Source: CAD feature listing. Evaluate the final solid. Frame: model axes, mm. A direction names the side the tool comes from. Give positions to 0.01 mm unless a question says otherwise; leave off trailing zeros. Loops run counter-clockwise (first coordinate to the right, second up) from the corner with the lowest first, then second, coordinate; pieces in that order, holes last. Notation, with made-up numbers: (-9, 50.25) - (3, 50.25) arc R21 ccw to (3, 85.25) - close; hole circle Ø11 at (87, -5.75). An arc over 180 degrees is marked (long way). Write each question's results on one line, items separated by ' | '. Start each with the question number.
(1) Contact query for flat-ended pins moving along their axis: pin 1 (5 mm diameter, centred on x = 3, z = -28, fed in from +Y); pin 2 (3 mm diameter, centred on y = -3, z = -29.5, fed in from +X); pin 3 (4 mm diameter, centred on y = -2, z = 7.5, fed in from +X); pin 4 (2 mm diameter, centred on x = -26.5, z = -17.5, fed in from +Y). Output: stop coordinate, or through.
(2) Pull-direction query (X, two-part tool) for faces 1 (the flat face through (11, -11, -29)), 2 (the cylindrical face through (-5.08, -7.6, -3.89)), 3 (the flat face through (-8.534, -17.535, 5.019)), 4 (the cylindrical face through (-8.67, -6.9, -39.05)); classes: pulls with the +X half, pulls with the -X half, needs draft (parallel to the pull), parting line crosses it, or undercut.
(3) Material intervals for line 1 along Z through (x, y) = (0, -5.25); line 2 along Z through (x, y) = (-1.5, -3.25); line 3 along X through (y, z) = (-9.5, -32), sorted ascending. Write a range as [from, to].
(4) Cut plane B-B on y = -10. Return the cut outline in (x, z), then the cut area to 3 significant figures.
(5) Reachability of faces 5 (the flat face through (-1, 0, -8)), 6 (the flat face through (11, -6, 24)), 7 (the flat face through (0, -18, -9.9)) from +Z, -Z, +X, -X, +Y, -Y: full face, straight path, thin tool, end or side. Return the list, or none.
(6) Cut plane A-A on x = 0. Return the cut outline in (y, z), then the cut area to 3 significant figures.
from build123d import *

# Parameters (mm, degrees)
F0_R          = 40
F1_DEPTH      = 20
F2_W          = 11
F2_H          = 10
F3_DEPTH      = 50
F3_DEPTH_BACK = 10
F4_R          = 6
F6_DEPTH      = 5
F7_R          = 6.4
F8_DEPTH      = 25


# Not quite as in the source:
# - a pattern or mirror of a feature is missing from the dataset's text; its kind, count and spacing are read off the source's solid


with BuildPart() as f1:
    # F0 (on Front) → F1 (new body)
    with BuildSketch(Plane.XZ):
        Circle(F0_R)
    extrude(amount=F1_DEPTH)

    # F2 (on Right) → F3 (cut, two sides)
    with BuildSketch(Plane.YZ) as f3_sk:
        with Locations((-5.5, 29)):
            Rectangle(F2_W, F2_H)
    f3 = extrude(amount=F3_DEPTH, mode=Mode.SUBTRACT) + extrude(f3_sk.sketch, amount=-F3_DEPTH_BACK, mode=Mode.SUBTRACT)

    # F3_copies: F3 across plane
    add(f3.mirror(Plane(origin=(0, 0, 0), x_dir=(-1, 0, 0), z_dir=(0, 0, -1))), mode=Mode.SUBTRACT)

    # F4
    f4_edges = [f1.edges().sort_by_distance(p)[0] for p in [
        (-40, -20, 0),
    ]]
    fillet(f4_edges, radius=F4_R)

    # F5 (on face) → F6 (cut)
    with BuildSketch(Plane.XZ.offset(20)):
        Polygon((-5.715767665, -9.9), (5.715767665, -9.9), (11.43153533, 0), (5.715767665, 9.9), (-5.715767665, 9.9), (-11.43153533, 0), align=None)
    extrude(amount=-F6_DEPTH, mode=Mode.SUBTRACT)

    # F7 (on face) → F8 (cut)
    with BuildSketch(Plane.XZ.offset(15)):
        Circle(F7_R)
    extrude(amount=-F8_DEPTH, mode=Mode.SUBTRACT)


solid = f1.part
Ans:
1) pin 1: y = -11 | pin 2: x = -10 | pin 3: x = 39.62 | pin 4: y = 0
2) face 1: needs draft | face 2: undercut | face 3: undercut | face 4: parting line crosses it
3) line 1: [-40, -34], [-24, -6.4], [6.4, 24], [34, 40] | line 2: [-39.97, -34], [-24, -6.22], [6.22, 24], [34, 39.97] | line 3: [-24, -10]
4) outline: (-10, -34) - (-10, -24) - (32, -24) arc R40 ccw to (32, 24) - (-10, 24) - (-10, 34) - (21.07, 34) arc R40 ccw (long way) to (21.07, -34) - close; hole circle Ø12.8 at (0, 0) | area: 4,150 mm^2
5) face 5: +Z, -Z, +X, -X, +Y | face 6: +X, +Y | face 7: -Y
6) outline: (-20, -34) arc R6 ccw to (-14, -40) - (0, -40) - (0, -34) - (-11, -34) - (-11, -24) - (0, -24) - (0, -6.4) - (-15, -6.4) - (-15, -9.9) - (-20, -9.9) - close; (-20, 9.9) - (-15, 9.9) - (-15, 6.4) - (0, 6.4) - (0, 24) - (-11, 24) - (-11, 34) - (0, 34) - (0, 40) - (-14, 40) arc R6 ccw to (-20, 34) - close | area: 1,070 mm^2
